Autodesk Inventor part; units mm, degrees
ref_plane "YZ Plane" through (0, 0, 0) normal (1, 0, 0) x (0, 1, 0)
ref_plane "XZ Plane" through (0, 0, 0) normal (0, 1, 0) x (-1, 0, 0)
ref_plane "XY Plane" through (0, 0, 0) normal (0, 0, 1) x (1, 0, 0)
ref_plane "작업 평면1" through (23.5, -8, -2) normal (1, 0, 0) x (0, 0, -1)
sketch "스케치1" plane through (23.5, -8, -2) normal (1, 0, 0) x (0, 0, -1)
  line L0 (0, 16) -> (-8.15, 16)
  line L1 (-8.15, 16) -> (-8.15, 10.6)
  line L2 (-8.15, 10.6) -> (-12.15, 10.6)
  line L3 (-13.15, 9.6) -> (-12.15, 10.6)
  line L4 (-13.15, 9.6) -> (-13.15, 6.4)
  line L5 (-12.15, 5.4) -> (-13.15, 6.4)
  line L6 (-12.15, 5.4) -> (-8.15, 5.4)
  line L7 (-8.15, 5.4) -> (-8.15, 0)
  line L8 (-8.15, 0) -> (0, 0)
  line L9 (0, 16) -> (9.35, 16)
  line L10 (9.35, 16) -> (9.35, 15)
  line L11 (0, 0) -> (9.35, 0)
  line L12 (9.35, 0) -> (9.35, 1)
  line L13 (0, 16) -> (-8.15, 16)
  line L14 (-8.15, 10.6) -> (-12.15, 10.6)
  line L15 (-8.15, 10.6) -> (-12.15, 10.6)
  line L16 (-12.15, 10.6) -> (-13.15, 9.6)
  line L17 (-13.15, 6.4) -> (-12.15, 5.4)
  line L18 (8.35, 14) -> (9.35, 14)
  line L19 (9.35, 14) -> (9.35, 15)
  line L20 (8.35, 2) -> (9.35, 2)
  line L21 (9.35, 2) -> (9.35, 1)
  line L22 (8.35, 14) -> (8.35, 2)
  point P0 (-2, 8)
  point P1 (4.35, 10.6)
  point P2 (4.35, 5.4)
  dimension "d1" = 9.35
  dimension "d13" = 9.35
sketch "스케치2" plane through (-23.5, 8, 6.15) normal (0, 0, 1) x (1, 0, 0)
  arc A0 (7.9209, -9.6) -> (7.9209, -6.4) centre (6, -8) ccw
  line L0 (39.0791, -9.6) -> (7.9209, -9.6)
  circle A1 centre (6, -8) radius 2.5
  circle A2 centre (41, -8) radius 2.5
  circle A3 centre (41, -8) radius 2.5
  point P0 (23.5, -8)
  point P1 (7.9209, -6.4)
extrude "돌출1" add sketch "스케치1" against normal up to surface (47 mm away)
extrude "돌출2" cut sketch "스케치2" along normal mid plane 50
sketch "스케치3" plane through (-15.5791, 1.6, 11.15) normal (0, 0, 1) x (1, 0, 0)
  line L0 (15.5791, -14.4593) -> (15.5791, 15.5737)
  line L1 (-7.9209, 4.4) -> (-7.9209, -7.6)
  line L2 (-7.9209, 4.4) -> (11.0791, 4.4)
  line L3 (11.0791, 4.4) -> (11.0791, -7.6)
  line L4 (11.0791, -7.6) -> (-7.9209, -7.6)
  line L5 (-7.9209, -7.6) -> (-7.9209, 4.4)
  line L6 (39.0791, 4.4) -> (39.0791, -7.6)
  line L7 (39.0791, 4.4) -> (20.0791, 4.4)
  line L8 (20.0791, 4.4) -> (20.0791, -7.6)
  line L9 (20.0791, -7.6) -> (39.0791, -7.6)
  line L10 (39.0791, -7.6) -> (39.0791, 4.4)
  point P0 (15.5791, -1.6)
  dimension "d9" = 19
extrude "돌출3" cut sketch "스케치3" against normal up to surface (5 mm away)
sketch "스케치4" plane through (-4.5, 1.6, 11.15) normal (0, 0, 1) x (1, 0, 0)
  line L0 (0.6181, -0.2528) -> (7.2489, -0.2528) construction
  line L1 (7.2489, -0.2528) -> (7.2489, -2.6222) construction
  line L2 (7.2489, -2.6222) -> (0.6181, -2.6222) construction
  line L3 (0.6181, -2.6222) -> (0.6181, -0.2528) construction
  line L4 (2.8925, -1.8707) -> (2.0321, -1.8707)
  line L5 (2.0321, -1.8707) -> (2.0321, -2.7311)
  line L6 (2.0321, -2.7311) -> (1.7481, -2.7311)
  line L7 (1.7481, -2.7311) -> (1.7481, -1.8707)
  line L8 (1.7481, -1.8707) -> (0.8877, -1.8707)
  line L9 (0.8877, -1.8707) -> (0.8877, -1.5969)
  line L10 (0.8877, -1.5969) -> (1.7481, -1.5969)
  line L11 (1.7481, -1.5969) -> (1.7481, -0.7365)
  line L12 (1.7481, -0.7365) -> (2.0321, -0.7365)
  line L13 (2.0321, -0.7365) -> (2.0321, -1.5969)
  line L14 (2.0321, -1.5969) -> (2.8925, -1.5969)
  line L15 (2.8925, -1.5969) -> (2.8925, -1.8707)
  spline S0 degree 2 poles (4.0308, -0.5472) (3.9382, -0.5472) (3.755, -0.5925) (3.6665, -0.6274) knots 0 0 0 1 2 2 2
  spline S1 degree 2 poles (3.6665, -0.6274) (3.5841, -0.6624) (3.4627, -0.7365) (3.4154, -0.7695) knots 0 0 0 1 2 2 2
  line L16 (3.4154, -0.7695) -> (3.3948, -0.7695)
  line L17 (3.3948, -0.7695) -> (3.3948, -0.4093)
  spline S2 degree 2 poles (3.3948, -0.4093) (3.5059, -0.3496) (3.8867, -0.2528) (4.0576, -0.2528) knots 0 0 0 1 2 2 2
  spline S3 degree 2 poles (4.0576, -0.2528) (4.2305, -0.2528) (4.4878, -0.3228) (4.5927, -0.3969) knots 0 0 0 1 2 2 2
  spline S4 degree 2 poles (4.5927, -0.3969) (4.7039, -0.4772) (4.8191, -0.7098) (4.8191, -0.8662) knots 0 0 0 1 2 2 2
  spline S5 degree 2 poles (4.8191, -0.8662) (4.8191, -1.0762) (4.5433, -1.3932) (4.3498, -1.4343) knots 0 0 0 1 2 2 2
  line L18 (4.3498, -1.4343) -> (4.3498, -1.459)
  spline S6 degree 2 poles (4.3498, -1.459) (4.4301, -1.4755) (4.6133, -1.5496) (4.6915, -1.6237) knots 0 0 0 1 2 2 2
  spline S7 degree 2 poles (4.6915, -1.6237) (4.7697, -1.6957) (4.8685, -1.9263) (4.8685, -2.093) knots 0 0 0 1 2 2 2
  spline S8 degree 2 poles (4.8685, -2.093) (4.8685, -2.2638) (4.7512, -2.5541) (4.6442, -2.6652) knots 0 0 0 1 2 2 2
  spline S9 degree 2 poles (4.6442, -2.6652) (4.533, -2.7805) (4.2181, -2.8999) (4.0184, -2.8999) knots 0 0 0 1 2 2 2
  spline S10 degree 2 poles (4.0184, -2.8999) (3.827, -2.8999) (3.4524, -2.8072) (3.3248, -2.7434) knots 0 0 0 1 2 2 2
  line L19 (3.3248, -2.7434) -> (3.3248, -2.3832)
  line L20 (3.3248, -2.3832) -> (3.3495, -2.3832)
  spline S11 degree 2 poles (3.3495, -2.3832) (3.4565, -2.4614) (3.8188, -2.6055) (3.9979, -2.6055) knots 0 0 0 1 2 2 2
  spline S12 degree 2 poles (3.9979, -2.6055) (4.1028, -2.6055) (4.3128, -2.5396) (4.3828, -2.4635) knots 0 0 0 1 2 2 2
  spline S13 degree 2 poles (4.3828, -2.4635) (4.4507, -2.3873) (4.5227, -2.2062) (4.5227, -2.0683) knots 0 0 0 1 2 2 2
  spline S14 degree 2 poles (4.5227, -2.0683) (4.5227, -1.9304) (4.4425, -1.7513) (4.3704, -1.6998) knots 0 0 0 1 2 2 2
  spline S15 degree 2 poles (4.3704, -1.6998) (4.2984, -1.6484) (4.1028, -1.6093) (3.9876, -1.6093) knots 0 0 0 1 2 2 2
  line L21 (3.9876, -1.6093) -> (3.8435, -1.6093)
  line L22 (3.8435, -1.6093) -> (3.8435, -1.3273)
  line L23 (3.8435, -1.3273) -> (3.9567, -1.3273)
  spline S16 degree 2 poles (3.9567, -1.3273) (4.1852, -1.3273) (4.4733, -1.1091) (4.4733, -0.9012) knots 0 0 0 1 2 2 2
  spline S17 degree 2 poles (4.4733, -0.9012) (4.4733, -0.8045) (4.3992, -0.6666) (4.3396, -0.6254) knots 0 0 0 1 2 2 2
  spline S18 degree 2 poles (4.3396, -0.6254) (4.2757, -0.5822) (4.1193, -0.5472) (4.0308, -0.5472) knots 0 0 0 1 2 2 2
  line L24 (5.7969, -2.8463) -> (5.3893, -2.8463)
  line L25 (5.3893, -2.8463) -> (5.3893, -2.3606)
  line L26 (5.3893, -2.3606) -> (5.7969, -2.3606)
  line L27 (5.7969, -2.3606) -> (5.7969, -2.8463)
  spline S19 degree 2 poles (7.8902, -1.5763) (7.8902, -2.2597) (7.4929, -2.8999) (7.0792, -2.8999) knots 0 0 0 1 2 2 2
  spline S20 degree 2 poles (7.0792, -2.8999) (6.6593, -2.8999) (6.2662, -2.2474) (6.2662, -1.5784) knots 0 0 0 1 2 2 2
  spline S21 degree 2 poles (6.2662, -1.5784) (6.2662, -0.8909) (6.6634, -0.2549) (7.0792, -0.2549) knots 0 0 0 1 2 2 2
  spline S22 degree 2 poles (7.0792, -0.2549) (7.4971, -0.2549) (7.8902, -0.9136) (7.8902, -1.5763) knots 0 0 0 1 2 2 2
  spline S23 degree 2 poles (7.4538, -2.3503) (7.5032, -2.2247) (7.5444, -1.8378) (7.5444, -1.5763) knots 0 0 0 1 2 2 2
  spline S24 degree 2 poles (7.5444, -1.5763) (7.5444, -1.3149) (7.5032, -0.93) (7.4518, -0.8003) knots 0 0 0 1 2 2 2
  spline S25 degree 2 poles (7.4518, -0.8003) (7.4003, -0.6707) (7.2212, -0.5369) (7.0792, -0.5369) knots 0 0 0 1 2 2 2
  spline S26 degree 2 poles (7.0792, -0.5369) (6.9372, -0.5369) (6.754, -0.6707) (6.7005, -0.8045) knots 0 0 0 1 2 2 2
  spline S27 degree 2 poles (6.7005, -0.8045) (6.649, -0.9341) (6.612, -1.3293) (6.612, -1.5784) knots 0 0 0 1 2 2 2
  spline S28 degree 2 poles (6.612, -1.5784) (6.612, -1.846) (6.6449, -2.2041) (6.6984, -2.3441) knots 0 0 0 1 2 2 2
  spline S29 degree 2 poles (6.6984, -2.3441) (6.7478, -2.4758) (6.931, -2.6179) (7.0792, -2.6179) knots 0 0 0 1 2 2 2
  spline S30 degree 2 poles (7.0792, -2.6179) (7.2192, -2.6179) (7.4024, -2.4841) (7.4538, -2.3503) knots 0 0 0 1 2 2 2
  point P0 (4.5, -1.6)
extrude "돌출4" cut sketch "스케치4" against normal blind 5
properties part number "Bearing Spacer_V2_3mm"
The listing builds one solid part. Answer for the finished solid, in the listing's coordinates (mm). A direction names the side the tool comes from. Round coordinates to 2 decimals unless told otherwise and drop trailing zeros. Write each loop counter-clockwise with the first axis right and the second up, starting at its lowest first coordinate (ties: lowest second). Pieces come first, ordered by that corner, then holes. Notation, with made-up numbers: M -3.5,64.25 L 51.5,64.25 A19 ccw 51.5,75.25 Z; hole C 14,38 d5. An arc over 180 degrees is marked long. Write each question's results on one line, items separated by ' | '. Start each with the question number.
Item 1: For faces 4 (the face through (0, -2.6, 8)), 5 (the face through (0, 6, -11)), 6 (the face through (-2.468, 0.4, 8.7)), 7 (the face through (-4.5, 0, 9)), determine the directions among +Z, -Z, +X, -X, +Y, -Y from which every point of the face is accessible in a straight line to the end or side of a thin tool.
Item 2: Flat-ended cylindrical pins translate along their axes: pin 1 Ø6 at (x, y) = (17.5, 0) entering from -Z; pin 2 Ø0.9 at (y, z) = (0, 8.5) entering from +X; pin 3 Ø2.5 at (y, z) = (1, 8) entering from -X. Find the tip coordinate at first contact, or state that the pin passes through.
Item 3: A cutting plane is placed at B-B on z = 9.5. State how many separate pieces and enclosed holes the cut face has, and give its area (3 significant figures).
Item 4: A cutting plane is placed at C-C on x = 6.5. Write down the section's boundary in (y, z), and give its area (3 significant figures).
Item 5: A cutting plane is placed at A-A on x = -17.5. Write down the section's boundary in (y, z).
Item 6: Straight lines are drawn through the part: L1, parallel to Y at x = -17.5, z = -6.25; L2, parallel to X at y = -1.25, z = -9.25; L3, parallel to Y at x = -2, z = 6.25. For each, find the intervals that lie inside material, in ascending order. Write a range as [from, to].
Item 7: A cutting plane is placed at D-D on z = 5.5. Write down the section's boundary in (x, y), and give its area (3 significant figures).
Item 8: For a pull along X with two mould halves and no side action, classify faces 1 (the face through (0, 0, -10.35)), 2 (the face through (-3, -0.271, 9)), 3 (the face through (23.5, 0, -2)) as pulls with the +X half, pulls with the -X half, needs draft (parallel to the pull), parting line crosses it, or undercut.
Check sheet entries:
1) face 4: +Z, +X, -X, -Y | face 5: -Z, +X, -X | face 6: +Z | face 7: +Z, -X, +Y, -Y
2) pin 1: z = -10.35 | pin 2: x = 4.5 | pin 3: x = -4.5
3) separate pieces: 2 | enclosed holes: 4 | area: 42.0 mm²
4) outline: M -8,-11.35 L -6,-11.35 L -6,-10.35 L 6,-10.35 L 6,-11.35 L 8,-11.35 L 8,6.15 L -8,6.15 Z | area: 268 mm²
5) outline: M -8,-11.35 L -6,-11.35 L -6,-10.35 L -2.5,-10.35 L -2.5,6.15 L -8,6.15 Z; M 2.5,-10.35 L 6,-10.35 L 6,-11.35 L 8,-11.35 L 8,6.15 L 2.5,6.15 Z
6) L1: [-8, -2.5], [2.5, 8] | L2: [-23.5, -19.67], [-15.33, 15.33], [19.67, 23.5] | L3: [-2.6, -0.27], [0, 2.6]
7) outline: M -23.5,-8 L 23.5,-8 L 23.5,8 L -23.5,8 Z; hole C -17.5,0 d5; hole C 17.5,0 d5 | area: 713 mm²
8) face 1: needs draft | face 2: undercut | face 3: pulls with the +X half
